Work out the finished part from the listing and answer in its coordinate system (mm). A direction names the side the tool comes from. Coordinates: 2 decimals unless noted, no trailing zeros. Write each loop counter-clockwise with the first axis right and the second up, starting at its lowest first coordinate (ties: lowest second). Pieces come first, ordered by that corner, then holes. Notation, with made-up numbers: M 27.25,24 L 52.25,24 A17 cw 52.25,57 Z; hole C 15,54.25 d3. An arc over 180 degrees is marked long. Use CSV: the item, a comma, the result in double quotes.
from build123d import *

# Parameters (mm, degrees)
F0_W      = 37
F0_H      = 29
F0_W_2    = 33
F0_H_2    = 25
F1_DEPTH  = 12
F2_DEPTH  = 2
F4_DEPTH  = 2
F6_DEPTH  = 1
F7_W      = 8.75
F7_H      = 4.75
F7_W_2    = 12.25
F8_DEPTH  = 2
F10_DEPTH = 1
F11_DEPTH = 1
F13_DEPTH = 3
F14_R     = 1.5
F15_W     = 3
F15_H     = 3.5
F16_DEPTH = 27
F17_DEPTH = 2
F18_DEPTH = 0.5
F19_DEPTH = 1.25
F20_DEPTH = 1.5


with BuildPart() as f1:
    # F0 (on Top) → F1 (new body)
    with BuildSketch(Plane.XY):
        Rectangle(F0_W, F0_H)
        Rectangle(F0_W_2, F0_H_2, mode=Mode.SUBTRACT)
    extrude(amount=F1_DEPTH)

    # F0 (on Top) → F2 (join)
    with BuildSketch(Plane.XY):
        Rectangle(F0_W_2, F0_H_2)
    extrude(amount=F2_DEPTH)

    # F3 (on face) → F4 (cut)
    with BuildSketch(Plane(origin=(16.5, 0, 0), x_dir=(0, -1, 0), z_dir=(-1, 0, 0))):
        Polygon((2.5, 2), (10, 2), (10, 12), (-5.5, 12), (-5.5, 7), (2.5, 7), align=None)
    extrude(amount=-F4_DEPTH, mode=Mode.SUBTRACT)

    # F5 (on face) → F6 (cut)
    with BuildSketch(Plane.XY.offset(2)):
        Polygon((15.5, -10), (16.5, -10), (18.5, -10), (18.5, -2.5), (16.5, -2.5), (15.5, -2.5), align=None)
    extrude(amount=-F6_DEPTH, mode=Mode.SUBTRACT)

    # F7 (on face) → F8 (cut)
    with BuildSketch(Plane.YZ.offset(-16.5)):
        with Locations((8.125, 4.375)):
            Rectangle(F7_W, F7_H)
        with Locations((-6.375, 4.375)):
            Rectangle(F7_W_2, F7_H)
    extrude(amount=-F8_DEPTH, mode=Mode.SUBTRACT)

    # F9 (on face) → F10 (cut)
    with BuildSketch(Plane.XY.offset(2)):
        Polygon((-18.5, 3.75), (-16.5, 3.75), (-15.5, 3.75), (-15.5, 12.5), (-18.5, 12.5), align=None)
        Polygon((-15.5, -0.25), (-16.5, -0.25), (-18.5, -0.25), (-18.5, -12.5), (-15.5, -12.5), align=None)
    extrude(amount=-F10_DEPTH, mode=Mode.SUBTRACT)

    # F11 (add): a face of the model
    f11_faces = [f1.faces().sort_by_distance(p)[0] for p in [
        (0, 0, 0),
    ]]
    extrude(f11_faces, amount=F11_DEPTH)

    # F12 (on face) → F13 (cut)
    with BuildSketch(Plane(origin=(0, 0, -1), x_dir=(1, 0, 0), z_dir=(0, 0, -1))):
        with BuildLine():
            ThreePointArc((5.25, 14.5), (8, 11.75), (10.75, 14.5))
            Line((10.75, 14.5), (8, 14.5))
            Line((8, 14.5), (5.25, 14.5))
        make_face()
        with BuildLine():
            Line((8, -14.5), (10.75, -14.5))
            ThreePointArc((10.75, -14.5), (8, -11.75), (5.25, -14.5))
            Line((5.25, -14.5), (8, -14.5))
        make_face()
    extrude(amount=-F13_DEPTH, mode=Mode.SUBTRACT)

    # F14
    f14_edges = [f1.edges().sort_by_distance(p)[0] for p in [
        (-18.5, -14.5, 5.5),
        (18.5, -14.5, 5.5),
        (18.5, 14.5, 5.5),
        (-18.5, 14.5, 5.5),
    ]]
    fillet(f14_edges, radius=F14_R)

    # F15 (on face) → F16 (cut)
    with BuildSketch(Plane.XZ.offset(-12.5)):
        with Locations((0, 10.25)):
            Rectangle(F15_W, F15_H)
    extrude(amount=F16_DEPTH, mode=Mode.SUBTRACT)

    # F15 (on face) → F17 (cut)
    with BuildSketch(Plane.XZ.offset(-12.5)):
        with Locations((0, 10.25)):
            Rectangle(F15_W, F15_H)
    extrude(amount=-F17_DEPTH, mode=Mode.SUBTRACT)

    # F18 (cut): a face of the model
    f18_faces = [f1.faces().sort_by_distance(p)[0] for p in [
        (17.5, 1.5, 7),
    ]]
    extrude(f18_faces, amount=-F18_DEPTH, mode=Mode.SUBTRACT)

    # F19 (cut): faces of the model
    f19_faces = [f1.faces().sort_by_distance(p)[0] for p in [
        (10.8712359215, -13.1995864394, 12),
        (9.25, 14.3076461594, 12),
        (-17.8229628853, -13.8229628853, 12),
    ]]
    extrude(f19_faces, amount=-F19_DEPTH, mode=Mode.SUBTRACT)

    # F20 (cut): faces of the model
    f20_faces = [f1.faces().sort_by_distance(p)[0] for p in [
        (0, -13.5, 8.5),
        (0, 13.5, 8.5),
    ]]
    extrude(f20_faces, amount=-F20_DEPTH, mode=Mode.SUBTRACT)


solid = f1.part
Item 1: For a pull along Y with two mould halves and no side action, classify faces 4 (the face through (8, -14, 2)), 5 (the face through (17, -10, 6)), 6 (the face through (-17, 3.75, 4)), 7 (the face through (0, 14.5, 5)) as released by +Y, released by -Y, zero draft, split by the parting line, or undercut.
Answer:
face 4,"zero draft"
face 5,"undercut"
face 6,"undercut"
face 7,"released by +Y"
Item 2: The part is cut by section B-B (y = 10.25). Write down the section's boundary in (x, z), then the cut area to 4 significant figures.
Answer:
outline,"M -18.5,-1 L 18.5,-1 L 18.5,10.75 L 16.5,10.75 L 16.5,2 L -15.5,2 L -15.5,1 L -18.5,1 Z; M -18.5,6.75 L -16.5,6.75 L -16.5,10.75 L -18.5,10.75 Z"
area,"133.5 mm2"
Item 3: The part is cut by section D-D (x = -0.5). Write down the section's boundary in (y, z).
Answer:
outline,"M -14.5,-1 L 14.5,-1 L 14.5,7 L 12.5,7 L 12.5,2 L -12.5,2 L -12.5,7 L -14.5,7 Z"
Item 4: Given pin 1 (1.6 mm diameter, centred on x = 0, y = 13.5, fed in from +Z); pin 2 (2.5 mm diameter, centred on x = 17.5, y = -8, fed in from +Z); pin 3 (1.6 mm diameter, centred on x = 17.5, y = 2.5, fed in from +Z), each flat-ended and moving along its own axis, determine where each tip first touches the part or whether it passes through.
Answer:
pin 1,"stops at z = 7"
pin 2,"stops at z = 1"
pin 3,"stops at z = 6.5"
Item 5: Consider probe 1 along X at (y, z) = (9.75, 10); probe 2 along Y at (x, z) = (-16, 5); probe 3 along Z at (x, y) = (3.5, -9). Determine where each line is inside the solid, lowest interval first.
Answer:
probe 1,"x = -18.5 to -16.5, 16.5 to 18.5"
probe 2,"y = -14.5 to -12.5, 12.5 to 14.5"
probe 3,"z = -1 to 2"
Item 6: A tool of negligible diameter and unlimited length cuts with its end or side. For faces 1 (the face through (-17, -6, 1)), 2 (the face through (17, -2.5, 4)), 3 (the face through (7.94, -11.75, 0.48)), from which of +Z, -Z, +X, -X, +Y, -Y can it reach the whole face along a straight path? Write none if from no direction.
Answer:
face 1,"-X"
face 2,"+Z, +X"
face 3,"-Z, -Y"
Item 7: The part is cut by section C-C (z = 0.5). Write down the section's boundary in (x, y), then the cut area to 3 significant figures.
Answer:
outline,"M -18.5,-13 A1.5 ccw -17,-14.5 L 5.25,-14.5 A2.75 cw 10.75,-14.5 L 17,-14.5 A1.5 ccw 18.5,-13 L 18.5,13 A1.5 ccw 17,14.5 L 10.75,14.5 A2.75 cw 5.25,14.5 L -17,14.5 A1.5 ccw -18.5,13 Z"
area,"1,050 mm2"
Item 8: The part is cut by section A-A (x = 8). Write down the section's boundary in (y, z).
Answer:
outline,"M -14.5,2 L -12.5,2 L -12.5,10.75 L -14.5,10.75 Z; M -11.75,-1 L 11.75,-1 L 11.75,2 L -11.75,2 Z; M 12.5,2 L 14.5,2 L 14.5,10.75 L 12.5,10.75 Z"
